The listing builds one solid part. Answer for the finished solid, in the listing's coordinates (mm). A direction names the side the tool comes from. Give positions to 0.01 mm unless a question says otherwise; leave off trailing zeros. Answer in a Markdown table with one row per item.
from build123d import *

# Parameters (mm, degrees)
F0_R     = 1.75
F1_DEPTH = 1.5
F2_SIZE  = 1.49999
F3_R     = 8


# Not quite as in the source:
# - a fillet or chamfer is up to 0.001 mm smaller than in the source, because OpenCascade refuses the exact size


with BuildPart() as f1:
    # F0 (on Top) → F1 (new body)
    with BuildSketch(Plane.XY):
        Polygon((0, 28.5), (0, 0), (8.5, 0), (8.5, 3), (17, 3), (17, 0), (28, 0), (28, 10), (8.6, 10), (8.6, 28.5), align=None)
        with Locations((4, 4.8)):
            Circle(F0_R, mode=Mode.SUBTRACT)
        with Locations((23, 4.8)):
            Circle(F0_R, mode=Mode.SUBTRACT)
        with Locations((4, 22.8)):
            Circle(F0_R, mode=Mode.SUBTRACT)
    extrude(amount=F1_DEPTH)

    # F2 (size 1.5 in the source; OpenCascade refuses exactly that, so slightly less here)
    f2_edges = [f1.edges().sort_by_distance(p)[0] for p in [
        (2.25, 22.8, 1.5),
        (2.25, 4.8, 1.5),
        (21.25, 4.8, 1.5),
    ]]
    chamfer(f2_edges, length=F2_SIZE)

    # F3
    f3_edges = [f1.edges().sort_by_distance(p)[0] for p in [
        (8.6, 10, 0.75),
    ]]
    fillet(f3_edges, radius=F3_R)


solid = f1.part
Item 1: Determine the mould class of faces 1 (the face through (13, 3, 1)), 2 (the face through (4, 0, 1)), 3 (the face through (28, 5, 1)) for opening direction X: pulls with the +X half, pulls with the -X half, needs draft (parallel to the pull), parting line crosses it, or undercut.
Answer block:
| item | result |
|---|---|
| face 1 | undercut |
| face 2 | needs draft |
| face 3 | pulls with the +X half |
Item 2: Find section C-C on y = 4.8. Count the separate pieces of the cut face and the enclosed holes in it, then the cut area to 3 significant figures.
Answer block:
| item | result |
|---|---|
| separate pieces | 3 |
| enclosed holes | 0 |
| area | 27.0 mm² |
Item 3: Consider line 1 (X direction, y = 5, z = 1); line 2 (Y direction, x = 4, z = 0.05); line 3 (X direction, y = 5.5, z = 1.25). Determine where each line is inside the solid, lowest interval first.
Answer block:
| item | result |
|---|---|
| line 1 | 0 to 1.26, 6.74 to 20.26, 25.74 to 28 |
| line 2 | 0 to 3, 6.6 to 21, 24.6 to 28.5 |
| line 3 | 0 to 1.08, 6.92 to 20.08, 25.92 to 28 |
Item 4: Each of these flat-tipped pins is pushed along its axis until it touches: P1, Ø3, axis at x = 23, y = 4.8, coming from the -Z side; P2, Ø5.5, axis at x = 4, y = 22.8, coming from the +Z side. Where does it stop, or does it pass through?
Answer block:
| item | result |
|---|---|
| P1 | through |
| P2 | z = 1 |
Item 5: Which of the six approach directions +Z, -Z, +X, -X, +Y, -Y give full straight-line access (tool end or side, diameter ignored) to faces 4 (the face through (22, 10, 1)), 5 (the face through (8.5, 1, 1)), 6 (the face through (11, 11, 0))?
Answer block:
| item | result |
|---|---|
| face 4 | +Z, -Z, +X, +Y |
| face 5 | +Z, -Z, -Y |
| face 6 | -Z, +X, -X, +Y, -Y |
